```python
from build123d import *

# Parameters (mm, degrees)
F1_DEPTH = 10
F2_DEPTH = 10
F3_R     = 1.75
F4_DEPTH = 25
F5_R     = 1.75
F6_DEPTH = 25


with BuildPart() as f1:
    # F0 (on Top) → F1 (new body)
    with BuildSketch(Plane.XY):
        with BuildLine():
            Line((10.976, -2.2287718591), (9.8, -1.9899748742))
            ThreePointArc((9.8, -1.9899748742), (-0.999999957, -9.9498743754), (-10, -8.64e-08))
            Line((-10, -8.64e-08), (-10, -5.0438080852))
            ThreePointArc((-10, -5.0438080852), (0.6909576709, -11.178666177), (10.5450266852, -3.7739120563))
            ThreePointArc((10.5450266852, -3.7739120563), (10.7882117125, -3.0090676374), (10.976, -2.2287718591))
        make_face()
        with BuildLine():
            Line((-10, 5), (-10, -8.64e-08))
            ThreePointArc((-10, -8.64e-08), (-4.32e-08, 10), (10, 0))
            Line((10, 0), (11.2, 0))
            ThreePointArc((11.2, 0), (11.1712443776, 0.8020592601), (11.0851251684, 1.6))
            ThreePointArc((11.0851251684, 1.6), (1.781171417, 11.0574603044), (-10.0219758531, 5))
            Line((-10.0219758531, 5), (-10, 5))
        make_face()
        with BuildLine():
            Line((-10, -5.0438080852), (-10, -8.64e-08))
            Line((-10, -8.64e-08), (-10, 5))
            Line((-10, 5), (-10.0219758531, 5))
            ThreePointArc((-10.0219758531, 5), (-11.199973191, -0.0245055425), (-10, -5.0438080852))
        make_face()
        with BuildLine():
            Line((20.776, -4.2187467333), (10.976, -2.2287718591))
            ThreePointArc((10.976, -2.2287718591), (10.7882117125, -3.0090676374), (10.5450266852, -3.7739120563))
            Line((10.5450266852, -3.7739120563), (20.4576040201, -5.7867467333))
            Line((20.4576040201, -5.7867467333), (20.776, -4.2187467333))
        make_face()
        with BuildLine():
            Line((-10, -15), (-10, -5.0438080852))
            ThreePointArc((-10, -5.0438080852), (-11.199973191, -0.0245055425), (-10.0219758531, 5))
            Line((-10.0219758531, 5), (-11.6, 5))
            Line((-11.6, 5), (-11.6, -15))
            Line((-11.6, -15), (-10, -15))
        make_face()
        with BuildLine():
            ThreePointArc((11.0851251684, 1.6), (11.1712443776, 0.8020592601), (11.2, 0))
            Line((11.2, 0), (21.2, 0))
            Line((21.2, 0), (21.2, 1.6))
            Line((21.2, 1.6), (11.0851251684, 1.6))
        make_face()
    extrude(amount=-F1_DEPTH)

    # F0 (on Top) → F2 (join)
    with BuildSketch(Plane.XY):
        with BuildLine():
            Line((-10, -15), (-10, -5.0438080852))
            ThreePointArc((-10, -5.0438080852), (-11.199973191, -0.0245055425), (-10.0219758531, 5))
            Line((-10.0219758531, 5), (-11.6, 5))
            Line((-11.6, 5), (-11.6, -15))
            Line((-11.6, -15), (-10, -15))
        make_face()
        with BuildLine():
            Line((-10, -5.0438080852), (-10, -8.64e-08))
            Line((-10, -8.64e-08), (-10, 5))
            Line((-10, 5), (-10.0219758531, 5))
            ThreePointArc((-10.0219758531, 5), (-11.199973191, -0.0245055425), (-10, -5.0438080852))
        make_face()
    extrude(amount=F2_DEPTH)

    # F3 (on face) → F4 (cut)
    with BuildSketch(Plane(origin=(-11.6, 0, 0), x_dir=(0, -1, 0), z_dir=(-1, 0, 0))):
        with Locations((0, 5)):
            Circle(F3_R)
        with BuildLine():
            ThreePointArc((11.75, 5), (10, 6.75), (8.25, 5))
            ThreePointArc((8.25, 5), (10, 3.25), (11.75, 5))
        make_face()
    extrude(amount=-F4_DEPTH, mode=Mode.SUBTRACT)

    # F5 (on face) → F6 (cut)
    with BuildSketch(Plane(origin=(0, 1.6, 0), x_dir=(-1, 0, 0), z_dir=(0, 1, 0))):
        with Locations((-16.1425625842, -5)):
            Circle(F5_R)
    extrude(amount=-F6_DEPTH, mode=Mode.SUBTRACT)


solid = f1.part
```
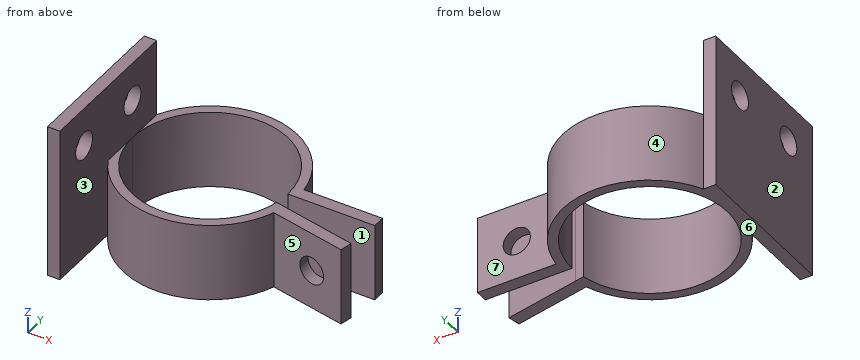
Geometry check sheet. Reference: the model listing, model coordinates, mm. Face numbers are marked on the shaded views. A direction names the side the tool comes from. Coordinates: 2 decimals unless noted, no trailing zeros. Write each loop counter-clockwise with the first axis right and the second up, starting at its lowest first coordinate (ties: lowest second). Pieces come first, ordered by that corner, then holes. Notation, with made-up numbers: M 83,48.5 L 123,48.5 A29 cw 123,74.5 Z; hole C 12,40 d7. An arc over 180 degrees is marked long. Use one line per item in the form item = value. Start each with the question number.
1) Section check D-D on y = -8.75. Enter the section's corners in (x, z), and give its area (3 significant figures).
2) Section check A-A on x = 0. Enter the section's corners in (y, z), and give its area (3 significant figures).
3) Set-up check for the marked faces 5, 6 and 7: record each of +Z, -Z, +X, -X, +Y, -Y from which the full face is reachable in a straight line by a thin tool's end or side.
4) Release check for a two-part mould opening along X. For the marked faces 1, 2, 3 and 4 record: pulls with the +X half, pulls with the -X half, needs draft (parallel to the pull), parting line crosses it, or undercut.
5) Section check B-B on z = 5. Enter the section's corners in (x, y).
6) Go/stop test with flat-tipped pins: pin 1 Ø12.5 at (x, y) = (5, 3.5) entering from +Z; pin 2 Ø5 at (x, z) = (17.5, -5) entering from -Y; pin 3 Ø4 at (y, z) = (-10, 5) entering from +X; pin 4 Ø3 at (x, z) = (16.14, -5) entering from -Y. Record where each tip stops, or that it passes through.
7) Thickness scan on probe 1 along Z at (x, y) = (-11.15, 0); probe 2 along X at (y, z) = (-7, -2.5); probe 3 along X at (y, z) = (0.25, -6.25). Record the ranges inside material, lowest first. Write a range as from..to.
Responses:
q1.outline = M -11.6,-10 L -10,-10 L -10,3.78 L -11.6,3.78 Z; M -11.6,6.22 L -10,6.22 L -10,10 L -11.6,10 Z; M -6.99,-10 L -4.84,-10 L -4.84,0 L -6.99,0 Z; M 4.84,-10 L 6.99,-10 L 6.99,0 L 4.84,0 Z
q1.area = 71.1 mm2
q2.outline = M -11.2,-10 L -10,-10 L -10,0 L -11.2,0 Z; M 10,-10 L 11.2,-10 L 11.2,0 L 10,0 Z
q2.area = 24.0 mm2
q3.face_5 = +Z, -Z, -Y
q3.face_6 = -Z, +X, -X, +Y, -Y
q3.face_7 = +Z, -Z, +X, +Y
q4.face_1 = needs draft
q4.face_2 = pulls with the -X half
q4.face_3 = undercut
q4.face_4 = parting line crosses it
q5.outline = M -11.6,-15 L -10,-15 L -10,-11.75 L -11.6,-11.75 Z; M -11.6,-8.25 L -10,-8.25 L -10,-1.75 L -11.6,-1.75 Z; M -11.6,1.75 L -10,1.75 L -10,5 L -11.6,5 Z
q6.pin_1 = 0
q6.pin_2 = -5.69
q6.pin_3 = -10
q6.pin_4 = through
q7.probe_1 = -10..3.25, 6.75..10
q7.probe_2 = -11.6..-10, -8.74..-7.14, 7.14..8.74
q7.probe_3 = -11.6..-10, 10..14.92, 17.37..21.2
